For this review, take the finished solid that the model builds, in its own axes (mm). Face numbers are marked on the shaded views. A direction names the side the tool comes from. Round coordinates to 2 decimals unless told otherwise and drop trailing zeros. Loops run counter-clockwise (first coordinate to the right, second up) from the corner with the lowest first, then second, coordinate; pieces in that order, holes last. Notation, with made-up numbers: M 79,28.25 L 132,28.25 A20 ccw 132,37.25 Z; hole C -15.5,-29.75 d5. An arc over 180 degrees is marked long. Write item = value, one per line. Start each with the question number.
```python
from build123d import *

# Parameters (mm, degrees)
CYLINDER_R              = 1.6
CYLINDER_DEPTH          = 22.6
CYLINDER001_R           = 3.1
CYLINDER001_DEPTH       = 25
CYLINDER002_R           = 5.8
CYLINDER002_DEPTH       = 25
CUBE002_W               = 22.6
CUBE002_H               = 1.1
CUBE002_DEPTH           = 11
CUBE003_W               = 22.6
CUBE003_H               = 1.1
CUBE003_DEPTH           = 11
CUBE004_W               = 30
CUBE004_H               = 3
CUBE004_DEPTH           = 8
CUBE004_PLACEMENT_ANGLE = 160
PRISM_DEPTH             = 2.5
CUBE005_W               = 22.6
CUBE005_H               = 6
CUBE005_DEPTH           = 6
CUBE005_PLACEMENT_ANGLE = 115
CUBE006_W               = 22.6
CUBE006_H               = 27
CUBE006_DEPTH           = 28
CUBE006_PLACEMENT_ANGLE = 45
CUBE007_W               = 22.6
CUBE007_H               = 10
CUBE007_DEPTH           = 10
CUBE007_PLACEMENT_ANGLE = 20
CYLINDER003_R           = 11
CYLINDER003_DEPTH       = 11.6
CUBE001_W               = 11.6
CUBE001_H               = 25
CUBE001_DEPTH           = 29
CUBE_W                  = 21.6
CUBE_H                  = 25
CUBE_DEPTH              = 28
SKETCH_W                = 9
SKETCH_H                = 8
POCKET_DEPTH            = 1
CHAMFER_SIZE            = 1


with BuildPart() as cylinder:
    # cylinder → cylinder (new body)
    with BuildSketch(Plane(origin=(-0.1, 20, 9), x_dir=(0, 0, -1), z_dir=(1, 0, 0))):
        Circle(CYLINDER_R)
    extrude(amount=CYLINDER_DEPTH)


with BuildPart() as cylinder001:
    # cylinder001 → cylinder001 (new body)
    with BuildSketch(Plane(origin=(10.8, -0.1, 18), x_dir=(1, 0, 0), z_dir=(0, 1, 0))):
        Circle(CYLINDER001_R)
    extrude(amount=CYLINDER001_DEPTH)


with BuildPart() as cylinder002:
    # cylinder002 → cylinder002 (new body)
    with BuildSketch(Plane(origin=(10.8, 4.4, 18), x_dir=(1, 0, 0), z_dir=(0, 1, 0))):
        Circle(CYLINDER002_R)
    extrude(amount=CYLINDER002_DEPTH)


with BuildPart() as cube002:
    # cube002 → cube002 (new body)
    with BuildSketch(Plane(origin=(-0.1, -0.1, 3), x_dir=(1, 0, 0), z_dir=(0, 0, 1))):
        with Locations((11.3, 0.55)):
            Rectangle(CUBE002_W, CUBE002_H)
    extrude(amount=CUBE002_DEPTH)


with BuildPart() as cube003:
    # cube003 → cube003 (new body)
    with BuildSketch(Plane(origin=(-0.1, -0.1, 22), x_dir=(1, 0, 0), z_dir=(0, 0, 1))):
        with Locations((11.3, 0.55)):
            Rectangle(CUBE003_W, CUBE003_H)
    extrude(amount=CUBE003_DEPTH)


with BuildPart() as cube004:
    # cube004 → cube004 (new body)
    with BuildSketch(Plane.XY):
        with Locations((15, 1.5)):
            Rectangle(CUBE004_W, CUBE004_H)
    extrude(amount=CUBE004_DEPTH)


with BuildPart() as cube004_1:
    # cube004 placement: moved
    add(cube004.part.moved(Location((-0.1, 1, 14))).rotate(Axis((-0.1, 1, 14), (1, 0, 0)), CUBE004_PLACEMENT_ANGLE))


with BuildPart() as prism:
    # prism → prism (new body)
    with BuildSketch(Plane(origin=(-0.1, 20, 9), x_dir=(0, 0, -1), z_dir=(1, 0, 0))):
        Polygon((3, 0), (1.5, 2.598076), (-1.5, 2.598076), (-3, 0), (-1.5, -2.598076), (1.5, -2.598076), align=None)
    extrude(amount=PRISM_DEPTH)


with BuildPart() as cube005:
    # cube005 → cube005 (new body)
    with BuildSketch(Plane.XY):
        with Locations((11.3, 3)):
            Rectangle(CUBE005_W, CUBE005_H)
    extrude(amount=CUBE005_DEPTH)


with BuildPart() as cube005_1:
    # cube005 placement: moved
    add(cube005.part.moved(Location((-0.1, 1, 0))).rotate(Axis((-0.1, 1, 0), (1, 0, 0)), CUBE005_PLACEMENT_ANGLE))


with BuildPart() as cube006:
    # cube006 → cube006 (new body)
    with BuildSketch(Plane.XY):
        with Locations((11.3, 13.5)):
            Rectangle(CUBE006_W, CUBE006_H)
    extrude(amount=CUBE006_DEPTH)


with BuildPart() as cube006_1:
    # cube006 placement: moved
    add(cube006.part.moved(Location((-0.1, 25, 13))).rotate(Axis((-0.1, 25, 13), (1, 0, 0)), CUBE006_PLACEMENT_ANGLE))


with BuildPart() as cube007:
    # cube007 → cube007 (new body)
    with BuildSketch(Plane.XY):
        with Locations((11.3, 5)):
            Rectangle(CUBE007_W, CUBE007_H)
    extrude(amount=CUBE007_DEPTH)


with BuildPart() as cube007_1:
    # cube007 placement: moved
    add(cube007.part.moved(Location((-0.1, 23, 0))).rotate(Axis((-0.1, 23, 0), (-1, 0, 0)), CUBE007_PLACEMENT_ANGLE))


with BuildPart() as cylinder003:
    # cylinder003 → cylinder003 (new body)
    with BuildSketch(Plane(origin=(5, 20, 9), x_dir=(0, 0, -1), z_dir=(1, 0, 0))):
        Circle(CYLINDER003_R)
    extrude(amount=CYLINDER003_DEPTH)


with BuildPart() as group:
    # cube001 → cube001 (new body)
    with BuildSketch(Plane(origin=(5, 8, -0.1), x_dir=(1, 0, 0), z_dir=(0, 0, 1))):
        with Locations((5.8, 12.5)):
            Rectangle(CUBE001_W, CUBE001_H)
    extrude(amount=CUBE001_DEPTH)

    # Group: union cylinder, cylinder001, cylinder002, cube002, cube003, cube004, prism, cube005, cube006, cube007, cylinder003
    add(cylinder.part)
    add(cylinder001.part)
    add(cylinder002.part)
    add(cube002.part)
    add(cube003.part)
    add(cube004_1.part)
    add(prism.part)
    add(cube005_1.part)
    add(cube006_1.part)
    add(cube007_1.part)
    add(cylinder003.part)


with BuildPart() as body:
    # cube → cube (new body)
    with BuildSketch(Plane.XY):
        with Locations((10.8, 12.5)):
            Rectangle(CUBE_W, CUBE_H)
    extrude(amount=CUBE_DEPTH)

    # difference: cut Group
    add(group.part, mode=Mode.SUBTRACT)

    # Sketch (on Face6 of BaseFeature) → Pocket (cut)
    with BuildSketch(Plane.XZ):
        with Locations((10.8, 18)):
            Rectangle(SKETCH_W, SKETCH_H)
    extrude(amount=-POCKET_DEPTH, mode=Mode.SUBTRACT)

    # Chamfer
    chamfer_edges = [body.edges().sort_by_distance(p)[0] for p in [
        (18.45, 0, 14.36397),
        (3.15, 0, 14.36397),
    ]]
    chamfer(chamfer_edges, length=CHAMFER_SIZE)


solid = body.part
```
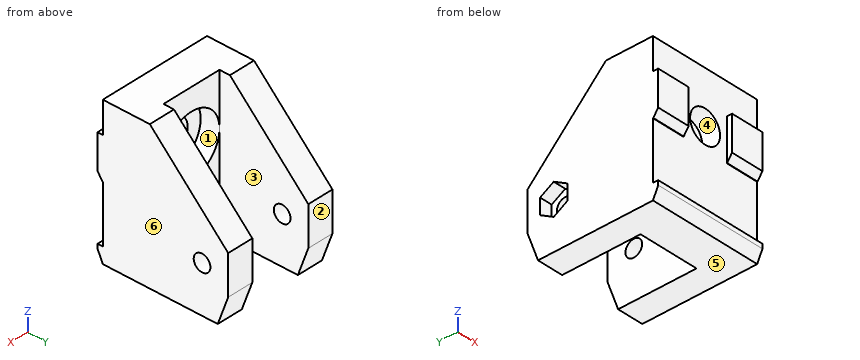
(1) Tool access review of the marked faces 1, 2 and 3: name each direction out of +Z, -Z, +X, -X, +Y, -Y from which nothing blocks a thin tool from reaching the whole face with its end or side.
(2) Add section A-A on y = 11.75. Write out the cut boundary in (x, z), and give its area (4 significant figures).
(3) Draft analysis for pull direction X (two halves, no side actions). For the marked faces 4, 5 and 6, state which applies: +X half, -X half, draft (parallel to the pull), parting line (faces both ways), or undercut.
(4) Wall thickness on L1, parallel to X at y = 12.5, z = 2.5; L2, parallel to Z at x = 4.25, y = 20; L3, parallel to Y at x = 19.3, z = 9: over which ranges is each line inside the solid? List them lowest first.
(5) Add section C-C on z = 9. Write out the cut boundary in (x, y), and give its area (3 significant figures).
(6) Add section B-B on x = 10.8. Write out the cut boundary in (y, z).
(7) Add section D-D on x = 19.75. Write out the cut boundary in (y, z), and give its area (3 significant figures).
(8) For pin 1 Ø0.5 at (x, y) = (18, 0.5) entering from +Z; pin 2 Ø4 at (x, z) = (10.5, 21.5) entering from +Y; pin 3 Ø3 at (y, z) = (20, 9) entering from -X; pin 4 Ø3.5 at (x, z) = (13, 12.5) entering from +Y, all flat-tipped, find the tip position at first contact; note any pin that passes through.
Answer sheet:
q1.face_1 = +Y
q1.face_2 = +Z, -Z, +X, -X, +Y
q1.face_3 = +Z, -Z, +Y
q2.outline = M 0,0 L 5,0 L 5,26.25 L 0,26.25 Z; M 16.6,0 L 21.6,0 L 21.6,26.25 L 16.6,26.25 Z
q2.area = 262.5 mm²
q3.face_4 = undercut
q3.face_5 = draft
q3.face_6 = +X half
q4.L1 = 0 to 5, 16.6 to 21.6
q4.L2 = 0 to 7.4, 10.6 to 18
q4.L3 = 1 to 18.4, 21.6 to 25
q5.outline = M 0,1 L 21.6,1 L 21.6,18.4 L 16.6,18.4 L 16.6,8 L 5,8 L 5,18.4 L 2.4,18.4 L 2.4,17.4 L 0,17.4 Z; M 0,22.6 L 2.4,22.6 L 2.4,21.6 L 5,21.6 L 5,25 L 0,25 Z; M 16.6,21.6 L 21.6,21.6 L 21.6,25 L 16.6,25 Z
q5.area = 284 mm²
q6.outline = M 0,2.14 L 1,0 L 8,0 L 8,12.2 L 4.4,12.2 L 4.4,14.9 L 1,14.9 L 1,3 L 0,3 Z; M 1,21.1 L 4.4,21.1 L 4.4,23.8 L 8,23.8 L 8,28 L 1,28 Z
q7.outline = M 0,2.14 L 1,0 L 23,0 L 25,5.49 L 25,13 L 10,28 L 1,28 L 1,22 L 0,22 L 0,15.36 L 0.94,14.02 L 1,14 L 1,3 L 0,3 Z; hole C 20,9 d3.2
q7.area = 555 mm²
q8.pin_1 = 22
q8.pin_2 = 4.4
q8.pin_3 = through
q8.pin_4 = 8
